from build123d import *

# Parameters (mm, degrees)
BOX004_W        = 16
BOX004_H        = 26
BOX004_DEPTH    = 14
SKETCH023_R     = 1.68
POCKET014_DEPTH = 19
SKETCH022_R     = 10.6
POCKET015_DEPTH = 10
SKETCH024_W     = 13
SKETCH024_H     = 10
POCKET016_DEPTH = 3
FILLET007_R     = 7.8


with BuildPart() as part:
    # Box004 → Box004 (new body)
    with BuildSketch(Plane(origin=(87, 12, -14), x_dir=(1, 0, 0), z_dir=(0, 0, 1))):
        with Locations((8, 13)):
            Rectangle(BOX004_W, BOX004_H)
    extrude(amount=BOX004_DEPTH)

    # Sketch023 → Pocket014 (cut)
    with BuildSketch(Plane(origin=(87, 12, -14), x_dir=(1, 0, 0), z_dir=(0, 0, -1))):
        with Locations((9, -5.2)):
            Circle(SKETCH023_R)
    extrude(amount=-POCKET014_DEPTH, mode=Mode.SUBTRACT)

    # Sketch022 → Pocket015 (cut)
    with BuildSketch(Plane(origin=(87, 12, 0), x_dir=(1, 0, 0), z_dir=(0, 0, 1))):
        with Locations((9, 5.2)):
            Circle(SKETCH022_R)
    extrude(amount=-POCKET015_DEPTH, mode=Mode.SUBTRACT)

    # Sketch024 → Pocket016 (cut)
    with BuildSketch(Plane(origin=(103, 12, -14), x_dir=(0, 1, 0), z_dir=(1, 0, 0))):
        with Locations((19.5, 9)):
            Rectangle(SKETCH024_W, SKETCH024_H)
    extrude(amount=-POCKET016_DEPTH, mode=Mode.SUBTRACT)

    # Fillet007
    fillet007_edges = [part.edges().sort_by_distance(p)[0] for p in [
        (87, 12, -12),
        (103, 12, -12),
    ]]
    fillet(fillet007_edges, radius=FILLET007_R)


solid = part.part
Geometry check sheet. Reference: the model listing, model coordinates, mm. A direction names the side the tool comes from. Give positions to 0.01 mm unless a question says otherwise; leave off trailing zeros. Write each loop counter-clockwise with the first axis right and the second up, starting at its lowest first coordinate (ties: lowest second). Pieces come first, ordered by that corner, then holes. Notation, with made-up numbers: (36, 69) - (60, 69) arc R21 ccw to (60, 78) - close; hole circle Ø1 at (71.25, 48.25). An arc over 180 degrees is marked (long way). Put each result on its own line as item: value.
1. Thickness scan on line 1 (Z direction, x = 91.75, y = 14.25); line 2 (X direction, y = 35.5, z = -9.5); line 3 (Y direction, x = 96, z = -11.9). Record the ranges inside material, lowest first.
Ans:
line 1: z = -14 to -10
line 2: x = 87 to 100
line 3: y = 12.04 to 15.52, 18.88 to 38
2. Go/stop test with flat-tipped pins: pin 1 (1 mm diameter, centred on x = 98.5, y = 22.5, fed in from +Z); pin 2 (5 mm diameter, centred on y = 34, z = -4.5, fed in from +X). Record where each tip stops, or that it passes through.
Ans:
pin 1: stops at z = -10
pin 2: stops at x = 100
3. Sectioned sample at B-B, the plane z = -10.5. Enter the section's corners in (x, y).
Ans:
outline: (87, 19.8) arc R7.8 ccw to (94.8, 12) - (95.2, 12) arc R7.8 ccw to (103, 19.8) - (103, 38) - (87, 38) - close; hole circle Ø3.36 at (96, 17.2)
4. Sectioned sample at C-C, the plane x = 96. Enter the section's corners in (y, z).
Ans:
outline: (12.04, -14) - (15.52, -14) - (15.52, -10) - (12.04, -10) - close; (18.88, -14) - (38, -14) - (38, 0) - (27.8, 0) - (27.8, -10) - (18.88, -10) - close
5. Sectioned sample at D-D, the plane y = 30.5. Enter the section's corners in (x, z), plus the area to 3 significant figures.
Ans:
outline: (87, -14) - (103, -14) - (103, -10) - (100, -10) - (100, 0) - (87, 0) - close
area: 194 mm²
6. Sectioned sample at A-A, the plane y = 17.2. Enter the section's corners in (x, z).
Ans:
outline: (87.45, -14) - (94.32, -14) - (94.32, -10) - (87.45, -10) - close; (97.68, -14) - (102.55, -14) - (102.55, -10) - (97.68, -10) - close
7. Draft check along X on faces 3 (the cylindrical face through (92.829, 27.315, -4.93)), 4 (the flat face through (95, 25, -14)), 5 (the flat face through (103, 29, -12)), 6 (the cylindrical face through (97.602, 16.695, -12.028)). Enter one of: +X half, -X half, draft (parallel to the pull), parting line (faces both ways), or undercut.
Ans:
face 3: undercut
face 4: draft
face 5: +X half
face 6: undercut
8. Set-up check for faces 1 (the flat face through (100, 32, -5)), 2 (the cylindrical face through (89.22, 14.35, -11.97)): record each of +Z, -Z, +X, -X, +Y, -Y from which the full face is reachable in a straight line by a thin tool's end or side.
Ans:
face 1: +Z, +X, +Y, -Y
face 2: +Z, -Z, -X, -Y
